The model under review builds one solid part; all positions refer to its coordinate system, in mm. Coordinates: 2 decimals unless noted, no trailing zeros. Order: outer loops, then holes, each group sorted by start corner. A loop starts at its lowest first (then second) coordinate and runs counter-clockwise, first axis right, second up. Notation, with made-up numbers: M 23,29.25 L 45,29.25 A34 ccw 45,63.25 Z; hole C 84,30 d8. An arc over 180 degrees is marked long. Answer in a Markdown table with one row per item.
from build123d import *

# Parameters (mm, degrees)
SKETCH1_W                                       = 50.8
SKETCH1_H                                       = 50.8
BOSS_EXTRUDE1_DEPTH                             = 2.54
FILLET1_R                                       = 1.5875
CSK_FOR_M3_FLAT_HEAD_MACHINE_SCREW1_D           = 3.175
CSK_FOR_M3_FLAT_HEAD_MACHINE_SCREW1_CSINK_D     = 5.588
CSK_FOR_M3_FLAT_HEAD_MACHINE_SCREW1_CSINK_ANGLE = 100
SKETCH4_W                                       = 13
SKETCH4_H                                       = 19.4
CUT_EXTRUDE1_DEPTH                              = 72.886936368
SKETCH5_R                                       = 1.4605
CUT_EXTRUDE2_DEPTH                              = 72.886936368


with BuildPart() as part:
    # Sketch1 → Boss-Extrude1 (new body)
    with BuildSketch(Plane(origin=(0, 0, 0), x_dir=(1, 0, 0), z_dir=(0, 1, 0))):
        with Locations((25.4, 25.4)):
            Rectangle(SKETCH1_W, SKETCH1_H)
    extrude(amount=BOSS_EXTRUDE1_DEPTH)

    # Fillet1
    fillet1_edges = [part.edges().sort_by_distance(p)[0] for p in [
        (50.8, 2.54, -25.4),
        (25.4, 2.54, -50.8),
        (0, 2.54, -25.4),
        (25.4, 2.54, 0),
    ]]
    fillet(fillet1_edges, radius=FILLET1_R)

    # CSK for M3 Flat Head Machine Screw1 (through all)
    with Locations(Plane(origin=(0, 2.54, 0), x_dir=(1, 0, 0), z_dir=(0, 1, 0))):
        with Locations((3.175, 47.625), (47.625, 47.625), (47.625, 3.175), (3.175, 3.175)):
            CounterSinkHole(CSK_FOR_M3_FLAT_HEAD_MACHINE_SCREW1_D / 2, CSK_FOR_M3_FLAT_HEAD_MACHINE_SCREW1_CSINK_D / 2, counter_sink_angle=CSK_FOR_M3_FLAT_HEAD_MACHINE_SCREW1_CSINK_ANGLE)

    # Sketch4 → Cut-Extrude1 (cut, through all)
    with BuildSketch(Plane(origin=(0, 2.54, 0), x_dir=(1, 0, 0), z_dir=(0, 1, 0))):
        with Locations((14.4375, 25.4)):
            Rectangle(SKETCH4_W, SKETCH4_H)
    extrude(amount=-CUT_EXTRUDE1_DEPTH, mode=Mode.SUBTRACT)

    # Sketch5 → Cut-Extrude2 (cut, through all)
    with BuildSketch(Plane(origin=(0, 2.54, 0), x_dir=(1, 0, 0), z_dir=(0, 1, 0))):
        with Locations(Location((38.1, 38.1, 0), (0, 0, 270))):
            Circle(SKETCH5_R)
    extrude(amount=-CUT_EXTRUDE2_DEPTH, mode=Mode.SUBTRACT)


solid = part.part
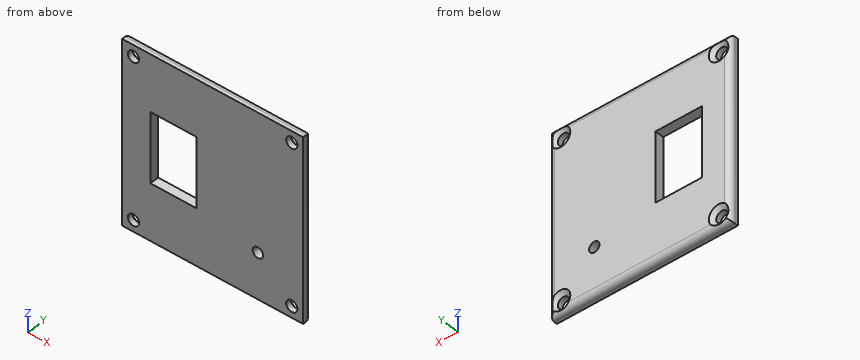
(1) Take a section at A-A (z = -33). Write out the cut boundary in (x, y) (1 decimal), then the cut area to 3 significant figures.
Report:
| item | result |
|---|---|
| outline | M 0,0 L 7.9,0 L 7.9,2.5 L 1.6,2.5 A1.6 ccw 0,1 Z; M 20.9,0 L 50.8,0 L 50.8,1 A1.6 ccw 49.2,2.5 L 20.9,2.5 Z |
| area | 94.9 mm^2 |
(2) Take a section at B-B (x = 18). Write out the cut boundary in (y, z) (1 decimal), then the cut area to 3 significant figures.
Report:
| item | result |
|---|---|
| outline | M 0,-50.8 L 1,-50.8 A1.6 ccw 2.5,-49.2 L 2.5,-35.1 L 0,-35.1 Z; M 0,-15.7 L 2.5,-15.7 L 2.5,-1.6 A1.6 ccw 1,0 L 0,0 Z |
| area | 78.7 mm^2 |
(3) Take a section at C-C (x = 48). State how many separate pieces and enclosed holes the cut face has, then the cut area to 3 significant figures.
Report:
| item | result |
|---|---|
| separate pieces | 3 |
| enclosed holes | 0 |
| area | 110 mm^2 |
(4) Insertion check: P1, Ø1, axis at x = 20, y = 2, coming from the +Z side. The pin has a flat end and moves straight along its axis. Give the tip position at first contact, or say it passes through.
Report:
| item | result |
|---|---|
| P1 | z = -0.1 |
(5) To check wall thickness, follow line 1 (Z direction, x = 15.5, y = 0.7); line 2 (X direction, y = 1.65, z = -3); line 3 (X direction, y = 0.5, z = -24). State the ranges of each line that lie inside material, in increasing order. Write a range as [from, to].
Report:
| item | result |
|---|---|
| line 1 | [-50.8, -35.1], [-15.7, 0] |
| line 2 | [0.16, 1.45], [4.9, 45.9], [49.35, 50.64] |
| line 3 | [0, 7.94], [20.94, 50.8] |
